from build123d import *

# Parameters (mm, degrees)
CROQUIS2_W              = 508
CROQUIS2_H              = 635
SALIENTE_EXTRUIR2_DEPTH = 38.1
CROQUIS3_R              = 19.05
CORTAR_EXTRUIR1_DEPTH   = 38.1
CROQUIS4_R              = 22.5
CORTAR_EXTRUIR2_DEPTH   = 38.1


with BuildPart() as part:
    # Croquis2 → Saliente-Extruir2 (new body)
    with BuildSketch(Plane(origin=(0, 0, 0), x_dir=(1, 0, 0), z_dir=(0, 1, 0))):
        Rectangle(CROQUIS2_W, CROQUIS2_H)
    extrude(amount=SALIENTE_EXTRUIR2_DEPTH)

    # Croquis3 → Cortar-Extruir1 (cut)
    with BuildSketch(Plane(origin=(0, 38.1, 0), x_dir=(1, 0, 0), z_dir=(0, 1, 0))):
        with Locations((-209.55, 273.05)):
            Circle(CROQUIS3_R)
        with Locations((209.55, 273.05)):
            Circle(CROQUIS3_R)
        with Locations((209.55, -273.05)):
            Circle(CROQUIS3_R)
        with Locations((-209.55, -273.05)):
            Circle(CROQUIS3_R)
    extrude(amount=-CORTAR_EXTRUIR1_DEPTH, mode=Mode.SUBTRACT)

    # Croquis4 → Cortar-Extruir2 (cut)
    with BuildSketch(Plane(origin=(0, 38.1, 0), x_dir=(1, 0, 0), z_dir=(0, 1, 0))):
        Circle(CROQUIS4_R)
    extrude(amount=-CORTAR_EXTRUIR2_DEPTH, mode=Mode.SUBTRACT)


solid = part.part
Check sheet for the modelled part. Datum: model origin and axes. Units: mm. Coordinates: 2 decimals unless noted, no trailing zeros. Loops run counter-clockwise (first coordinate to the right, second up) from the corner with the lowest first, then second, coordinate; pieces in that order, holes last. Notation, with made-up numbers: (8.25, 30.25) -> (41.25, 30.25) arc R33 cw to (41.25, 58.25) -> close; hole circle Ø9 at (6, 4). An arc over 180 degrees is marked (long way). Write item = value, one per line. Start each with the question number.
1. Draft check along Z on faces 1 (the flat face through (-4, 19, -317.5)), 2 (the flat face through (-254, 19, 4)), 3 (the cylindrical face through (190.52, 19.32, 272.21)), 4 (the cylindrical face through (-228.58, 19.32, 272.21)). Enter one of: released by +Z, released by -Z, zero draft, split by the parting line, or undercut.
2. Section check D-D on x = -209.55. Record the cut outline in (y, z), then the cut area to 3 significant figures.
3. Material ranges on line 1 (Z direction, x = -209.55, y = 10.5); line 2 (X direction, y = 21, z = 273.05); line 3 (X direction, y = 18, z = -271.5), recorded low to high.
4. Section check C-C on z = -273.05. Record the cut outline in (x, y), then the cut area to 3 significant figures.
5. Section check A-A on x = 0. Record the cut outline in (y, z), then the cut area to 3 significant figures.
6. Section check B-B on z = 0. Record the cut outline in (x, y).
7. Depth check by flat-ended pin: P1, Ø23, axis at x = 209.55, z = 273.05, coming from the +Y side. Enter the tip coordinate at first touch or a pass-through.
Responses:
q1.face_1 = released by -Z
q1.face_2 = zero draft
q1.face_3 = undercut
q1.face_4 = undercut
q2.outline = (0, -317.5) -> (38.1, -317.5) -> (38.1, -292.1) -> (0, -292.1) -> close; (0, -254) -> (38.1, -254) -> (38.1, 254) -> (0, 254) -> close; (0, 292.1) -> (38.1, 292.1) -> (38.1, 317.5) -> (0, 317.5) -> close
q2.area = 21,300 mm2
q3.line_1 = -317.5 to -292.1, -254 to 254, 292.1 to 317.5
q3.line_2 = -254 to -228.6, -190.5 to 190.5, 228.6 to 254
q3.line_3 = -254 to -228.54, -190.56 to 190.56, 228.54 to 254
q4.outline = (-254, 0) -> (-228.6, 0) -> (-228.6, 38.1) -> (-254, 38.1) -> close; (-190.5, 0) -> (190.5, 0) -> (190.5, 38.1) -> (-190.5, 38.1) -> close; (228.6, 0) -> (254, 0) -> (254, 38.1) -> (228.6, 38.1) -> close
q4.area = 16,500 mm2
q5.outline = (0, -317.5) -> (38.1, -317.5) -> (38.1, -22.5) -> (0, -22.5) -> close; (0, 22.5) -> (38.1, 22.5) -> (38.1, 317.5) -> (0, 317.5) -> close
q5.area = 22,500 mm2
q6.outline = (-254, 0) -> (-22.5, 0) -> (-22.5, 38.1) -> (-254, 38.1) -> close; (22.5, 0) -> (254, 0) -> (254, 38.1) -> (22.5, 38.1) -> close
q7.P1 = through
